```python
from build123d import *

# Parameters (mm, degrees)
SKETCH1_R           = 1.2
BOSS_EXTRUDE1_DEPTH = 7
SKETCH2_R           = 2.05
CUT_EXTRUDE1_DEPTH  = 2
FILLET1_R           = 0.5


with BuildPart() as part:
    # Sketch1 → Boss-Extrude1 (new body)
    with BuildSketch(Plane(origin=(0, 0, 0), x_dir=(1, 0, 0), z_dir=(0, 1, 0))):
        with BuildLine():
            Line((0, 0), (0, -5.17))
            Line((0, -5.17), (18, -5.17))
            Line((18, -5.17), (18, 0))
            ThreePointArc((18, 0), (9, 2.577794898), (0, 0))
        make_face()
        with Locations(Location((4, -0.17, 0), (0, 0, 270))):
            Circle(SKETCH1_R, mode=Mode.SUBTRACT)
        with Locations(Location((14, -0.17, 0), (0, 0, 270))):
            Circle(SKETCH1_R, mode=Mode.SUBTRACT)
    extrude(amount=BOSS_EXTRUDE1_DEPTH)

    # Sketch2 → Cut-Extrude1 (cut)
    with BuildSketch(Plane(origin=(0, 7, 0), x_dir=(1, 0, 0), z_dir=(0, 1, 0))):
        with Locations((4, -0.17)):
            Circle(SKETCH2_R)
        with Locations((14, -0.17)):
            Circle(SKETCH2_R)
    extrude(amount=-CUT_EXTRUDE1_DEPTH, mode=Mode.SUBTRACT)

    # Fillet1
    fillet1_edges = [part.edges().sort_by_distance(p)[0] for p in [
        (0, 7, 2.585),
        (9, 7, 5.17),
        (9, 7, -2.577794898),
        (1.271083669, 7, -0.719256266),
        (13.841338508, 6, -1.873850907),
        (15.400788894, 6, -1.326759992),
        (2.599211106, 6, -1.326759992),
        (4.158661492, 6, -1.873850907),
        (4.678636308, 7, 2.104412769),
        (13.321363692, 7, 2.104412769),
        (18, 7, 2.585),
        (9, 0, 5.17),
        (0, 0, 2.585),
        (9, 0, -2.577794898),
        (18, 0, 2.585),
        (18, 3.5, 5.17),
        (0, 3.5, 5.17),
        (0, 3.5, 0),
        (18, 3.5, 0),
        (16.728916331, 7, -0.719256266),
    ]]
    fillet(fillet1_edges, radius=FILLET1_R)


solid = part.part
```
Design review of the part built by this model. Coordinates are the model's own, in mm. A direction names the side the tool comes from. Round coordinates to 2 decimals unless told otherwise and drop trailing zeros. Order: outer loops, then holes, each group sorted by start corner. A loop starts at its lowest first (then second) coordinate and runs counter-clockwise, first axis right, second up. Notation, with made-up numbers: (48.5, 38) - (92.5, 38) arc R17 cw to (92.5, 46) - close; hole circle Ø1 at (1.25, -39). An arc over 180 degrees is marked (long way). Return JSON: item names as keys, results as strings.
Q1. For pin 1 Ø3 at (y, z) = (4, 1) entering from -X; pin 2 Ø1.3 at (x, z) = (4.5, 0.5) entering from +Y; pin 3 Ø1 at (x, y) = (2, 3.5) entering from -Z, all flat-tipped, find the tip position at first contact; note any pin that passes through.
Computed values:
{"pin 1": "stops at x = 0", "pin 2": "stops at y = 5", "pin 3": "stops at z = -1.29"}
Q2. Consider section A-A on y = 4.5. Write out the cut boundary in (x, z), plus the area to 3 significant figures.
Computed values:
{"outline": "(0, 0.28) arc R0.5 ccw to (0.24, -0.15) arc R17 ccw to (17.76, -0.15) arc R0.5 ccw to (18, 0.28) - (18, 4.67) arc R0.5 ccw to (17.5, 5.17) - (0.5, 5.17) arc R0.5 ccw to (0, 4.67) - close; hole circle Ø2.4 at (4, 0.17); hole circle Ø2.4 at (14, 0.17)", "area": "115 mm2"}
Q3. The part is to be moulded in two halves that separate along X. For faces 3 (the cylindrical face through (9.129, 3.458, -2.577)), 4 (the flat face through (5, 5, -1)), 5 (the flat face through (18, 3, 3)), 6 (the flat face through (9, 7, 2)), say which applies: pulls with the +X half, pulls with the -X half, needs draft (parallel to the pull), parting line crosses it, or undercut.
Computed values:
{"face 3": "parting line crosses it", "face 4": "undercut", "face 5": "pulls with the +X half", "face 6": "needs draft"}
Q4. Machinability: for faces 1 (the cylindrical face through (12.83, 2.46, -0.09)), 2 (the cylindrical face through (13.265, 5.76, 2.084)), which of the approach directions +Z, -Z, +X, -X, +Y, -Y give a long, thin tool a straight path to every point of the face, cutting with its end or side? Answer none if there is none.
Computed values:
{"face 1": "+Y, -Y", "face 2": "+Y"}
Q5. Wall thickness on L1, parallel to X at y = 6, z = 0.25; L2, parallel to X at y = 1, z = 0.25; L3, parallel to Z at x = 4, y = 3.5: over which ranges is each line inside the solid? List them lowest first. Write a range as [from, to].
Computed values:
{"L1": "x = [0, 1.95], [6.05, 11.95], [16.05, 18]", "L2": "x = [0, 2.8], [5.2, 12.8], [15.2, 18]", "L3": "z = [-1.83, -1.03], [1.37, 5.17]"}
